Input: part model. Units: mm. Frame: model coordinates. A direction names the side the tool comes from. Coordinates: 2 decimals unless noted, no trailing zeros. Loops run counter-clockwise (first coordinate to the right, second up) from the corner with the lowest first, then second, coordinate; pieces in that order, holes last. Notation, with made-up numbers: (33, 19.25) -> (72, 19.25) arc R36 ccw to (72, 56.25) -> close; hole circle Ø2 at (73.5, -6). An arc over 180 degrees is marked (long way). Answer as a JSON object with one key per item and string values.
from build123d import *

# Parameters (mm, degrees)
SKETCH_1_R           = 120
SKETCH_1_R_2         = 3
SKETCH_1_W           = 100
SKETCH_1_H           = 100
EXTRUDE_3_DEPTH      = 69
SKETCH_8_R           = 150
SKETCH_8_R_2         = 99.33727818
EXTRUDE_6_DEPTH      = 20
SKETCH_9_R           = 5
CUT_EXTRUDE_11_DEPTH = 10
CUT_EXTRUDE_12_DEPTH = 76


with BuildPart() as part:
    # 草图1 → 凸台-拉伸3 (new body)
    with BuildSketch(Plane(origin=(0, 0, 0), x_dir=(1, 0, 0), z_dir=(0, 1, 0))):
        with Locations(Location((-30.656096769, -1.474017122, 0), (0, 0, 270))):
            Circle(SKETCH_1_R)
        with Locations(Location((-90.656096769, -1.474017122, 0), (0, 0, 270))):
            Circle(SKETCH_1_R_2, mode=Mode.SUBTRACT)
        with Locations(Location((29.343903231, -1.474017122, 0), (0, 0, 270))):
            Circle(SKETCH_1_R_2, mode=Mode.SUBTRACT)
        with Locations(Location((-30.656096769, -61.474017122, 0), (0, 0, 270))):
            Circle(SKETCH_1_R_2, mode=Mode.SUBTRACT)
        with Locations(Location((-30.656096769, 58.525982878, 0), (0, 0, 270))):
            Circle(SKETCH_1_R_2, mode=Mode.SUBTRACT)
        with Locations((-30.656096769, -1.474017122)):
            Rectangle(SKETCH_1_W, SKETCH_1_H, mode=Mode.SUBTRACT)
    extrude(amount=EXTRUDE_3_DEPTH)

    # 草图8 → 凸台-拉伸6 (add)
    with BuildSketch(Plane(origin=(0, 69, 0), x_dir=(1, 0, 0), z_dir=(0, 1, 0))):
        with Locations(Location((-30.656096769, -1.474017122, 0), (0, 0, 270))):
            Circle(SKETCH_8_R)
        with Locations(Location((-30.656096769, -1.474017122, 0), (0, 0, 270))):
            Circle(SKETCH_8_R_2, mode=Mode.SUBTRACT)
    extrude(amount=EXTRUDE_6_DEPTH)

    # 草图9 → 切除-拉伸11 (cut)
    with BuildSketch(Plane(origin=(0, 89, 0), x_dir=(1, 0, 0), z_dir=(0, 1, 0))):
        with Locations(Location((-26.787702046, 125, 0), (0, 0, 270))):
            Circle(SKETCH_9_R)
        with Locations(Location((98.212297954, 0, 0), (0, 0, 270))):
            Circle(SKETCH_9_R)
        with Locations(Location((-26.787702046, -125, 0), (0, 0, 270))):
            Circle(SKETCH_9_R)
        with Locations(Location((-151.787702046, 0, 0), (0, 0, 270))):
            Circle(SKETCH_9_R)
    extrude(amount=-CUT_EXTRUDE_11_DEPTH, mode=Mode.SUBTRACT)

    # 草图10 → 切除-拉伸12 (cut)
    with BuildSketch(Plane(origin=(0, 0, 51.474017122), x_dir=(-1, 0, 0), z_dir=(0, 0, -1))):
        with BuildLine():
            Line((55.656096769, 21.899366297), (5.656196663, 21.899366297))
            ThreePointArc((5.656196663, 21.899366297), (-4.343803337, 31.899366297), (5.656196663, 41.899366297))
            Line((5.656196663, 41.899366297), (55.656096769, 41.899366297))
            ThreePointArc((55.656096769, 41.899366297), (65.656096769, 31.899366297), (55.656096769, 21.899366297))
        make_face()
    extrude(amount=-CUT_EXTRUDE_12_DEPTH, mode=Mode.SUBTRACT)


solid = part.part
1. Line query: line 1 along X through (y, z) = (85, 0); line 2 along Z through (x, y) = (-26.5, 53.5); line 3 along Z through (x, y) = (-14, 17). Output: solid intervals per line, ascending.
Reply:
{"line 1": "x = -180.65 to -156.79, -146.79 to -129.98, 68.67 to 93.21, 103.21 to 119.34", "line 2": "z = -118.45 to -48.53, 51.47 to 121.4", "line 3": "z = -117.36 to -48.53, 51.47 to 120.31"}
2. Section query C-C (z = -67). Return loops of the section in (x, y).
Reply:
{"outline": "(-164.12, 69) -> (-129.2, 69) -> (-129.2, 0) -> (67.89, 0) -> (67.89, 69) -> (102.8, 69) -> (102.8, 89) -> (41.31, 89) -> (41.31, 69) -> (-102.62, 69) -> (-102.62, 89) -> (-164.12, 89) -> close"}
3. Section query B-B (x = 39). Return loops of the section in (y, z), plus the area to 3 significant figures.
Reply:
{"outline": "(0, -96.24) -> (69, -96.24) -> (69, -131.37) -> (89, -131.37) -> (89, -69.35) -> (69, -69.35) -> (69, 72.3) -> (89, 72.3) -> (89, 134.32) -> (69, 134.32) -> (69, 99.19) -> (0, 99.19) -> close", "area": "16,000 mm2"}
4. Section query A-A (y = 63). Return loops of the section in (x, z), plus the area to 3 significant figures.
Reply:
{"outline": "circle Ø240 at (-30.66, 1.47); hole circle Ø6 at (-90.66, 1.47); hole (-80.66, -48.53) -> (19.34, -48.53) -> (19.34, 51.47) -> (-80.66, 51.47) -> close; hole circle Ø6 at (-30.66, -58.53); hole circle Ø6 at (-30.66, 61.47); hole circle Ø6 at (29.34, 1.47)", "area": "35,100 mm2"}
5. Section query D-D (z = 92). Return loops of the section in (x, y), plus the area to 3 significant figures.
Reply:
{"outline": "(-150.26, 69) -> (-109.43, 69) -> (-109.43, 0) -> (48.12, 0) -> (48.12, 69) -> (88.95, 69) -> (88.95, 89) -> (10.25, 89) -> (10.25, 69) -> (-71.56, 69) -> (-71.56, 89) -> (-150.26, 89) -> close; hole (-55.66, 21.9) -> (-5.66, 21.9) arc R10 ccw to (-5.66, 41.9) -> (-55.66, 41.9) arc R10 ccw to start", "area": "12,700 mm2"}
6. Pin query (flat end, axial travel): P1, Ø9, axis at x = -26.79, z = 125, coming from the +Y side; P2, Ø20.5, axis at x = -21, y = 28.5, coming from the -Z side; P3, Ø7, axis at x = -30.66, z = -58.53, coming from the -Y side; P4, Ø10, axis at y = 77.5, z = -101.5, coming from the +X side. Return the tip coordinate at first contact, or that it passes through.
Reply:
{"P1": "stops at y = 79", "P2": "stops at z = -118.53", "P3": "stops at y = 0", "P4": "stops at x = 82.93"}
7. Mould query, pull axis Y, two halves, no side actions, for faces 1 (the face through (-30, 41.899, 86)), 2 (the face through (-156.67, 84.07, -1.08)), 3 (the face through (-29, 69, 66)). Classes: pulls with the +Y half, pulls with the -Y half, needs draft (parallel to the pull), parting line crosses it, or undercut.
Reply:
{"face 1": "undercut", "face 2": "needs draft", "face 3": "pulls with the +Y half"}
8. Access query for faces 4 (the face through (70, 69, -66)), 5 (the face through (-29, 0, 53)), 6 (the face through (-152, 79, 0)), 7 (the face through (-31, 34, -48.526)), 8 (the face through (-31, 21.899, 86)). Directions: +Z, -Z, +X, -X, +Y, -Y. A direction counts if a zero-diameter tool reaches every point of the face in a straight line with its end or side. Return the directions, or none.
Reply:
{"face 4": "-Y", "face 5": "+Z, -Z, +X, -X, -Y", "face 6": "+Y", "face 7": "+Y, -Y", "face 8": "+Z"}
